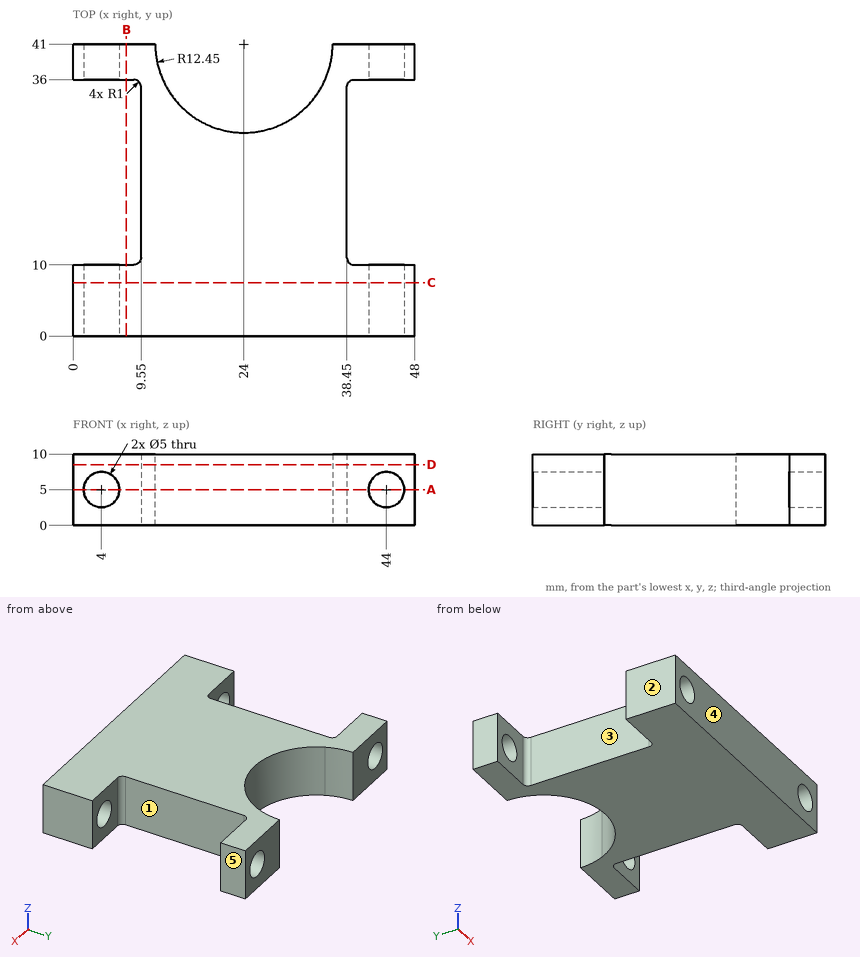
For this review, use the dimensioned drawing (mm, ordinates from the lowest corner) and the shaded views. A direction names the side the tool comes from. Give positions to 0.01 mm unless a question says otherwise; leave off trailing zeros. Order: outer loops, then holes, each group sorted by start corner. A loop starts at its lowest first (then second) coordinate and runs counter-clockwise, first axis right, second up. Notation, with made-up numbers: (-13.5, -15) - (19.5, -15) arc R36 ccw to (19.5, 20) - close; hole circle Ø9 at (40.5, 22). An arc over 180 degrees is marked (long way). Write item = value, one per line. Start each with the question number.
Q1. We need section D-D on z = 8.5. State the section outline as (x, y) points, plus the area to 3 significant figures.
Q2. Mouldability with a two-part tool opening along Y and no side actions: class the marked faces 3, 4 and 5 as released by +Y, released by -Y, zero draft, split by the parting line, or undercut.
Q3. We need section C-C on y = 7.5. State the section outline as (x, z) points, plus the area to 3 significant figures.
Q4. We need section A-A on z = 5. State how many separate pieces and enclosed holes the cut face has, plus the area to 3 significant figures.
Q5. Clearance check with flat-ended pins moving along their axes: pin 1 Ø2.5 at (x, z) = (2.5, 3) entering from -Y; pin 2 Ø5 at (y, z) = (21.5, 3.5) entering from -X; pin 3 Ø6 at (x, z) = (27, 4.5) entering from +Y; pin 4 Ø5 at (y, z) = (18.5, 5) entering from +X. State where each tip first meets the part, or that it passes through.
Q6. Tool access review of the marked faces 1 and 2: name each direction out of +Z, -Z, +X, -X, +Y, -Y from which nothing blocks a thin tool from reaching the whole face with its end or side.
Q7. We need section B-B on x = 7.5. State the section outline as (y, z) points.
Q8. To check wall thickness, follow L1, parallel to X at y = 5.25, z = 5; L2, parallel to X at y = 38.3, z = 5; L3, parallel to X at y = 37.2, z = 5. State the ranges of each line that lie inside material, in increasing order. Write a range as from..to.
Working result:
q1.outline = (0, 0) - (48, 0) - (48, 10) - (39.45, 10) arc R1 cw to (38.45, 11) - (38.45, 35) arc R1 cw to (39.45, 36) - (48, 36) - (48, 41) - (36.45, 41) arc R12.45 cw to (11.55, 41) - (0, 41) - (0, 36) - (8.55, 36) arc R1 cw to (9.55, 35) - (9.55, 11) arc R1 cw to (8.55, 10) - (0, 10) - close
q1.area = 1,230 mm²
q2.face_3 = undercut
q2.face_4 = released by -Y
q2.face_5 = zero draft
q3.outline = (0, 0) - (48, 0) - (48, 10) - (0, 10) - close; hole circle Ø5 at (4, 5); hole circle Ø5 at (44, 5)
q3.area = 441 mm²
q4.separate_pieces = 5
q4.enclosed_holes = 0
q4.area = 1,080 mm²
q5.pin_1 = 0
q5.pin_2 = 9.55
q5.pin_3 = 30.09
q5.pin_4 = 38.45
q6.face_1 = +Z, -Z, +X
q6.face_2 = +Z, -Z, -X, +Y, -Y
q7.outline = (0, 0) - (10, 0) - (10, 10) - (0, 10) - close; (36, 0) - (41, 0) - (41, 10) - (36, 10) - close
q8.L1 = 0..1.5, 6.5..41.5, 46.5..48
q8.L2 = 0..1.5, 6.5..11.85, 36.15..41.5, 46.5..48
q8.L3 = 0..1.5, 6.5..12.14, 35.86..41.5, 46.5..48
